Part print with two shaded views. Sizes in mm from the minimum x, y, z corner. A direction names the side the tool comes from. Coordinates: 2 decimals unless noted, no trailing zeros. Order: outer loops, then holes, each group sorted by start corner. A loop starts at its lowest first (then second) coordinate and runs counter-clockwise, first axis right, second up. Notation, with made-up numbers: M -0.5,-37.5 L 21.5,-37.5 A20 cw 21.5,-14.5 Z; hole C 22,-39 d6. An arc over 180 degrees is marked long. Answer in a Markdown table with one row per item. Add a question column.
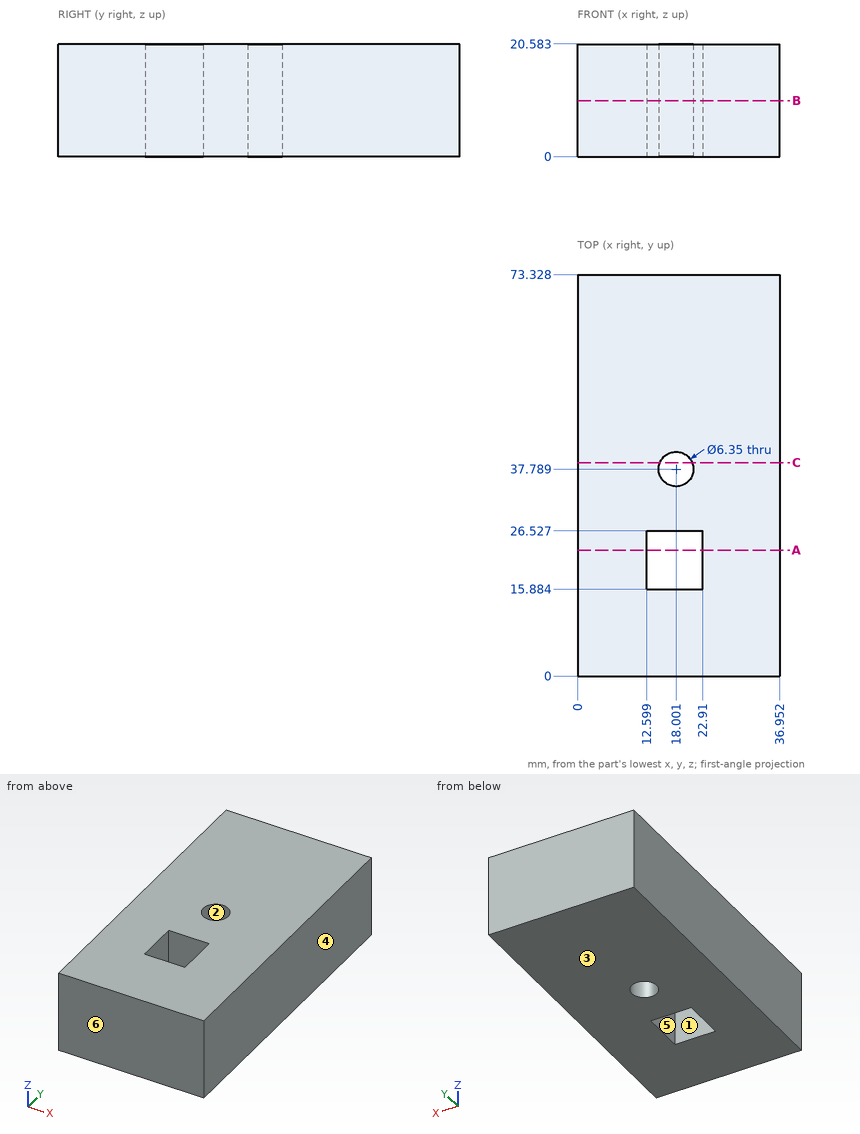
(1) Slice it at C-C (y = 39). List the corners of the cut face in (x, z).
(2) Pull direction X, two halves, no side cores. Call the marked faces 1, 2, 3 and 4: pulls with the +X half, pulls with the -X half, needs draft (parallel to the pull), parting line crosses it, or undercut.
(3) Wall check: line 1 (X direction, y = 23, z = 15.25); line 2 (Y direction, x = 17.5, z = 17.75) (1 decimal); line 3 (Y direction, x = 16, z = 3) (1 decimal). Give the ranges that are in metal, low to high.
(4) 3-axis set-ups, long thin cutter, end or side, ignore diameter. For the marked faces 5 and 6: which of +Z, -Z, +X, -X, +Y, -Y reach the whole face in a straight line?
(5) Slice it at A-A (y = 23). List the corners of the cut face in (x, z).
(6) Slice it at B-B (z = 10.25). State how many separate pieces and enclosed holes the cut face has, and give its area (3 significant figures).
Computed:
| question | item | result |
|---|---|---|
| 1 | outline | M 0,0 L 15.07,0 L 15.07,20.58 L 0,20.58 Z; M 20.94,0 L 36.95,0 L 36.95,20.58 L 20.94,20.58 Z |
| 2 | face 1 | undercut |
| 2 | face 2 | undercut |
| 2 | face 3 | needs draft |
| 2 | face 4 | pulls with the +X half |
| 3 | line 1 | x = 0 to 12.6, 22.91 to 36.95 |
| 3 | line 2 | y = 0 to 15.9, 26.5 to 34.7, 40.9 to 73.3 |
| 3 | line 3 | y = 0 to 15.9, 26.5 to 35.3, 40.3 to 73.3 |
| 4 | face 5 | +Z, -Z |
| 4 | face 6 | +Z, -Z, +X, -X, -Y |
| 5 | outline | M 0,0 L 12.6,0 L 12.6,20.58 L 0,20.58 Z; M 22.91,0 L 36.95,0 L 36.95,20.58 L 22.91,20.58 Z |
| 6 | separate pieces | 1 |
| 6 | enclosed holes | 2 |
| 6 | area | 2,570 mm^2 |
